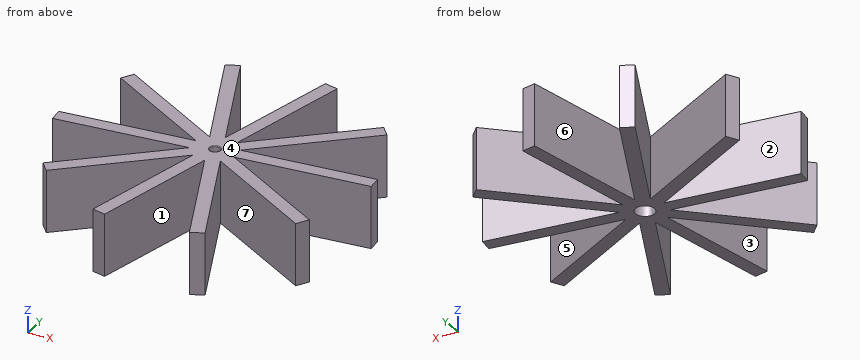
from build123d import *

# Parameters (mm, degrees)
F0_R      = 0.9525
F1_DEPTH  = 3.81
F2_R      = 0.127
F3_DEPTH  = 2.54
F4_DEPTH  = 24.13
F5_DEPTH  = 24.13
F6_DEPTH  = 24.13
F7_DEPTH  = 24.13
F8_DEPTH  = 24.13
F9_DEPTH  = 24.13
F10_DEPTH = 24.13
F11_DEPTH = 24.13
F12_DEPTH = 24.13
F13_DEPTH = 24.13
F14_DEPTH = 5.08
F15_R     = 1.778
F16_DEPTH = 5.08


with BuildPart() as f1:
    # F0 (on Top) → F1 (new body)
    with BuildSketch(Plane.XY):
        Polygon((0.4323873163, -4.0869975888), (2.7520855959, -3.0522996175), (4.0205807178, -0.8517269361), (3.75335066, 1.6741764857), (2.0524682218, 3.5606013931), (-0.4323873163, 4.0869975888), (-2.7520855959, 3.0522996175), (-4.0205807178, 0.8517269361), (-3.75335066, -1.6741764857), (-2.0524682218, -3.5606013931), align=None)
        Circle(F0_R, mode=Mode.SUBTRACT)
    extrude(amount=F1_DEPTH)

    # F2
    f2_edges = [f1.edges().sort_by_distance(p)[0] for p in [
        (-0.9525, 0, 3.81),
    ]]
    fillet(f2_edges, radius=F2_R)

    # F0 (on Top) → F3 (join)
    with BuildSketch(Plane.XY):
        Polygon((0.4323873163, -4.0869975888), (2.7520855959, -3.0522996175), (4.0205807178, -0.8517269361), (3.75335066, 1.6741764857), (2.0524682218, 3.5606013931), (-0.4323873163, 4.0869975888), (-2.7520855959, 3.0522996175), (-4.0205807178, 0.8517269361), (-3.75335066, -1.6741764857), (-2.0524682218, -3.5606013931), align=None)
        Circle(F0_R, mode=Mode.SUBTRACT)
        Circle(F0_R)
    extrude(amount=-F3_DEPTH)

    # F4 (add): a face of the model
    f4_faces = [f1.faces().sort_by_distance(p)[0] for p in [
        (2.9029094409, 2.6173889394, 0.635),
    ]]
    extrude(f4_faces, amount=F4_DEPTH)

    # F5 (add): a face of the model
    f5_faces = [f1.faces().sort_by_distance(p)[0] for p in [
        (3.8869656889, 0.4112247748, 0.635),
    ]]
    extrude(f5_faces, amount=F5_DEPTH)

    # F6 (add): a face of the model
    f6_faces = [f1.faces().sort_by_distance(p)[0] for p in [
        (3.3863331568, -1.9520132768, 0.635),
    ]]
    extrude(f6_faces, amount=F6_DEPTH)

    # F7 (add): a face of the model
    f7_faces = [f1.faces().sort_by_distance(p)[0] for p in [
        (1.5922364561, -3.5696486031, 0.635),
    ]]
    extrude(f7_faces, amount=F7_DEPTH)

    # F8 (add): a face of the model
    f8_faces = [f1.faces().sort_by_distance(p)[0] for p in [
        (-0.8100404527, -3.8237994909, 0.635),
    ]]
    extrude(f8_faces, amount=F8_DEPTH)

    # F9 (add): a face of the model
    f9_faces = [f1.faces().sort_by_distance(p)[0] for p in [
        (-2.9029094409, -2.6173889394, 0.635),
    ]]
    extrude(f9_faces, amount=F9_DEPTH)

    # F10 (add): a face of the model
    f10_faces = [f1.faces().sort_by_distance(p)[0] for p in [
        (-3.8869656889, -0.4112247748, 0.635),
    ]]
    extrude(f10_faces, amount=F10_DEPTH)

    # F11 (add): a face of the model
    f11_faces = [f1.faces().sort_by_distance(p)[0] for p in [
        (-3.3863331568, 1.9520132768, 0.635),
    ]]
    extrude(f11_faces, amount=F11_DEPTH)

    # F12 (add): a face of the model
    f12_faces = [f1.faces().sort_by_distance(p)[0] for p in [
        (-1.5922364561, 3.5696486031, 0.635),
    ]]
    extrude(f12_faces, amount=F12_DEPTH)

    # F13 (add): a face of the model
    f13_faces = [f1.faces().sort_by_distance(p)[0] for p in [
        (0.8100404527, 3.8237994909, 0.635),
    ]]
    extrude(f13_faces, amount=F13_DEPTH)

    # F14 (add): a face of the model
    f14_faces = [f1.faces().sort_by_distance(p)[0] for p in [
        (0, 0, -2.54),
    ]]
    extrude(f14_faces, amount=F14_DEPTH)

    # F15 (on face) → F16 (cut)
    with BuildSketch(Plane(origin=(0, 0, -7.62), x_dir=(1, 0, 0), z_dir=(0, 0, -1))):
        Circle(F15_R)
    extrude(amount=-F16_DEPTH, mode=Mode.SUBTRACT)


solid = f1.part
Source: CAD feature listing. Evaluate the final solid. Frame: model axes, mm. Face numbers are marked on the shaded views. A direction names the side the tool comes from. Give positions to 0.01 mm unless a question says otherwise; leave off trailing zeros. Write each loop counter-clockwise with the first axis right and the second up, starting at its lowest first coordinate (ties: lowest second). Pieces come first, ordered by that corner, then holes. Notation, with made-up numbers: M 86.25,-9 L 95.25,-9 A18 cw 95.25,26 Z; hole C -14.75,33.25 d7. An arc over 180 degrees is marked long. Return JSON: item names as keys, results as strings. Group by question number.
1) Pull-direction query (X, two-part tool) for the marked faces 1, 2, 3 and 4; classes: pulls with the +X half, pulls with the -X half, needs draft (parallel to the pull), parting line crosses it, or undercut.
2) Pin query (flat end, axial travel): P1, Ø5.5, axis at x = 0, y = 0, coming from the -Z side; P2, Ø6, axis at x = 11, z = -2.5, coming from the -Y side; P3, Ø3, axis at x = 12, z = -5, coming from the -Y side; P4, Ø1.1, axis at x = 0.5, y = -0.5, coming from the -Z side. Return the tip coordinate at first contact, or that it passes through.
3) Cut plane C-C, the plane x = 17. Output: boundary loops of the cut face in (y, z).
4) Cut plane B-B, the plane y = 7. Output: boundary loops of the cut face in (x, z).
5) Cut plane D-D, the plane y = 0. Output: boundary loops of the cut face in (x, z), plus the area to 3 significant figures.
6) Set-up query: the marked faces 5, 6 and 7. Return all of +Z, -Z, +X, -X, +Y, -Y with unobstructed straight access to the full face (end or side cutting, diameter ignored); none if empty.
7) Material intervals for line 1 along Y through (x, z) = (-11, -7); line 2 along Y through (x, z) = (13, 2.5); line 3 along Y through (x, z) = (-13.5, 2), sorted ascending. Write a range as [from, to].
Recorded:
{
 "1": {"face 1": "undercut", "face 2": "pulls with the -X half", "face 3": "undercut", "face 4": "needs draft"},
 "2": {"P1": "stops at z = -7.62", "P2": "stops at y = -26.12", "P3": "stops at y = -26.02", "P4": "stops at z = -2.54"},
 "3": {"outline": "M -11.27,-7.62 L -8.33,-7.62 L -8.33,3.81 L -11.27,3.81 Z; M 0.52,-7.62 L 3.08,-7.62 L 3.08,3.81 L 0.52,3.81 Z; M 13.62,-7.62 L 17.04,-7.62 L 17.04,3.81 L 13.62,3.81 Z"},
 "4": {"outline": "M -14.69,-7.62 L -9.6,-7.62 L -9.6,3.81 L -14.69,3.81 Z; M -4.51,-7.62 L -1.73,-7.62 L -1.73,3.81 L -4.51,3.81 Z; M 0.18,-7.62 L 2.78,-7.62 L 2.78,3.81 L 0.18,3.81 Z; M 5.87,-7.62 L 9.66,-7.62 L 9.66,3.81 L 5.87,3.81 Z"},
 "5": {"outline": "M -12.07,-7.62 L -1.78,-7.62 L -1.78,-2.54 L 1.78,-2.54 L 1.78,-7.62 L 12.07,-7.62 L 12.07,3.81 L 1.08,3.81 A0.13 ccw 0.95,3.68 L 0.95,0 L -0.95,0 L -0.95,3.68 A0.13 ccw -1.08,3.81 L -12.07,3.81 Z", "area": "251 mm²"},
 "6": {"face 5": "+Z, -Z, +X", "face 6": "+Z, -Z, +Y", "face 7": "+Z, -Z"},
 "7": {"line 1": "y = [-11.63, -8.21], [-2.44, 0.11], [4.87, 7.81], [21.54, 25.79]", "line 2": "y = [-8.96, -6.03], [0.1, 2.65], [10.01, 13.43]", "line 3": "y = [-13.88, -10.46], [-2.71, -0.15], [6.32, 9.25]"}
}
